The listing builds one solid part. Answer for the finished solid, in the listing's coordinates (mm). A direction names the side the tool comes from. Coordinates: 2 decimals unless noted, no trailing zeros. Order: outer loops, then holes, each group sorted by start corner. A loop starts at its lowest first (then second) coordinate and runs counter-clockwise, first axis right, second up. Notation, with made-up numbers: (32.5, 55.5) -> (85.5, 55.5) arc R26 ccw to (85.5, 93.5) -> close; hole circle Ø1 at (43, 2). An arc over 180 degrees is marked (long way). Return JSON: item names as keys, results as strings.
```python
from build123d import *

# Parameters (mm, degrees)
EXTRUDE_1_OUTLINE_R   = 35
EXTRUDE_1_OUTLINE_R_2 = 1.55
EXTRUDE_1_OUTLINE_R_3 = 30.05
EXTRUDE_1_DEPTH       = 10
SKETCH_2_R            = 33.525
SKETCH_2_R_2          = 18.525
EXTRUDE_1_2_DEPTH     = 4
SKETCH_3_R            = 1.55
CUT_EXTRUDE_1_DEPTH   = 51.497524692
CUT_EXTRUDE_2_DEPTH   = 6
SKETCH_8_R            = 35
SKETCH_8_R_2          = 30.05
CUT_EXTRUDE_3_DEPTH   = 2
SKETCH_9_R            = 3
CUT_EXTRUDE_4_DEPTH   = 2
SKETCH_10_R           = 1.55
CUT_EXTRUDE_5_DEPTH   = 51.139804547
SKETCH_11_R           = 3
CUT_EXTRUDE_6_DEPTH   = 2
SKETCH_14_R           = 18.525
SKETCH_14_R_2         = 13.5
EXTRUDE_2_DEPTH       = 4
SKETCH_15_R           = 17.5
CUT_EXTRUDE_8_DEPTH   = 1
SKETCH_17_R           = 17.5
SKETCH_17_R_2         = 12.5
CUT_EXTRUDE_9_DEPTH   = 1
SKETCH1_R             = 13.5
SKETCH1_R_2           = 12
BOSS_EXTRUDE1_DEPTH   = 1
SKETCH2_R             = 12.5
SKETCH2_R_2           = 12
CUT_EXTRUDE1_DEPTH    = 50.989999


# Read off the part's stored shape, not the designer's step: 凸台-拉伸1
with BuildPart() as part:
    # Extrude 1 outline → Extrude 1 (new body)
    with BuildSketch(Plane.XY):
        Circle(EXTRUDE_1_OUTLINE_R)
        with Locations((0, -32.5)):
            Circle(EXTRUDE_1_OUTLINE_R_2, mode=Mode.SUBTRACT)
        with Locations((-32.5, 0)):
            Circle(EXTRUDE_1_OUTLINE_R_2, mode=Mode.SUBTRACT)
        Circle(EXTRUDE_1_OUTLINE_R_3, mode=Mode.SUBTRACT)
        with Locations((32.5, 0)):
            Circle(EXTRUDE_1_OUTLINE_R_2, mode=Mode.SUBTRACT)
        with Locations((0, 32.5)):
            Circle(EXTRUDE_1_OUTLINE_R_2, mode=Mode.SUBTRACT)
    extrude(amount=EXTRUDE_1_DEPTH)

    # 草图2 → Extrude 1 2 (add)
    with BuildSketch(Plane.XY.offset(10)):
        Circle(SKETCH_2_R)
        Circle(SKETCH_2_R_2, mode=Mode.SUBTRACT)
    extrude(amount=-EXTRUDE_1_2_DEPTH)

    # 草图3 → 切除-拉伸1 (cut, through all)
    with BuildSketch(Plane(origin=(0, 0, 0), x_dir=(-1, 0, 0), z_dir=(0, 0, -1))):
        with Locations(Location((32.5, 0, 0), (0, 0, 180))):
            Circle(SKETCH_3_R)
        with Locations(Location((0, -32.5, 0), (0, 0, 180))):
            Circle(SKETCH_3_R)
        with Locations(Location((-32.5, 0, 0), (0, 0, 180))):
            Circle(SKETCH_3_R)
        with Locations(Location((0, 32.5, 0), (0, 0, 180))):
            Circle(SKETCH_3_R)
    extrude(amount=-CUT_EXTRUDE_1_DEPTH, mode=Mode.SUBTRACT)

    # 草图7 → 切除-拉伸2 (cut)
    with BuildSketch(Plane(origin=(0, 0, 0), x_dir=(-1, 0, 0), z_dir=(0, 0, -1))):
        with BuildLine():
            Line((15.025, 26.024063384), (17.5, 30.310889132))
            ThreePointArc((17.5, 30.310889132), (24.748737342, 24.748737342), (30.310889132, 17.5))
            Line((30.310889132, 17.5), (26.024063384, 15.025))
            ThreePointArc((26.024063384, 15.025), (21.248558775, 21.248558775), (15.025, 26.024063384))
        make_face()
    extrude(amount=-CUT_EXTRUDE_2_DEPTH, mode=Mode.SUBTRACT)

    # 草图8 → 切除-拉伸3 (cut)
    with BuildSketch(Plane(origin=(0, 0, 0), x_dir=(-1, 0, 0), z_dir=(0, 0, -1))):
        with Locations(Location((0, 0, 0), (0, 0, 30))):
            Circle(SKETCH_8_R)
        Circle(SKETCH_8_R_2, mode=Mode.SUBTRACT)
    extrude(amount=-CUT_EXTRUDE_3_DEPTH, mode=Mode.SUBTRACT)

    # 草图9 → 切除-拉伸4 (cut)
    with BuildSketch(Plane.XY.offset(10)):
        with Locations((0, 32.5)):
            Circle(SKETCH_9_R)
        with Locations((32.5, 0)):
            Circle(SKETCH_9_R)
        with Locations((0, -32.5)):
            Circle(SKETCH_9_R)
        with Locations((-32.5, 0)):
            Circle(SKETCH_9_R)
    extrude(amount=-CUT_EXTRUDE_4_DEPTH, mode=Mode.SUBTRACT)

    # 草图10 → 切除-拉伸5 (cut, through all)
    with BuildSketch(Plane.XY.offset(10)):
        with Locations((22.980970389, 22.980970389)):
            Circle(SKETCH_10_R)
        with Locations((22.980970389, -22.980970389)):
            Circle(SKETCH_10_R)
        with Locations((-22.980970389, -22.980970389)):
            Circle(SKETCH_10_R)
        with Locations((-22.980970389, 22.980970389)):
            Circle(SKETCH_10_R)
    extrude(amount=-CUT_EXTRUDE_5_DEPTH, mode=Mode.SUBTRACT)

    # 草图11 → 切除-拉伸6 (cut)
    with BuildSketch(Plane.XY.offset(10)):
        with Locations((22.980970389, 22.980970389)):
            Circle(SKETCH_11_R)
        with Locations((22.980970389, -22.980970389)):
            Circle(SKETCH_11_R)
        with Locations((-22.980970389, -22.980970389)):
            Circle(SKETCH_11_R)
        with Locations((-22.980970389, 22.980970389)):
            Circle(SKETCH_11_R)
    extrude(amount=-CUT_EXTRUDE_6_DEPTH, mode=Mode.SUBTRACT)

    # 草图14 → 凸台-拉伸2 (add)
    with BuildSketch(Plane.XY.offset(10)):
        Circle(SKETCH_14_R)
        Circle(SKETCH_14_R_2, mode=Mode.SUBTRACT)
    extrude(amount=-EXTRUDE_2_DEPTH)

    # 草图15 → 切除-拉伸8 (cut)
    with BuildSketch(Plane.XY.offset(10)):
        with BuildLine():
            ThreePointArc((21.378493867, 1.75), (0, 21.45), (-21.378493867, 1.75))
            Line((-21.378493866, 1.75), (-24.8, 1.75))
            Line((-24.8, 1.75), (-24.8, -1.75))
            Line((-24.8, -1.75), (-21.378493867, -1.75))
            ThreePointArc((-21.378493867, -1.75), (0, -21.45), (21.378493867, -1.75))
            Line((21.378493867, -1.75), (24.8, -1.75))
            Line((24.8, -1.75), (24.8, 1.75))
            Line((24.8, 1.75), (21.378493867, 1.75))
        make_face()
        Circle(SKETCH_15_R, mode=Mode.SUBTRACT)
    extrude(amount=-CUT_EXTRUDE_8_DEPTH, mode=Mode.SUBTRACT)

    # 草图17 → 切除-拉伸9 (cut)
    with BuildSketch(Plane.XY.offset(10)):
        Circle(SKETCH_17_R)
        Circle(SKETCH_17_R_2, mode=Mode.SUBTRACT)
    extrude(amount=-CUT_EXTRUDE_9_DEPTH, mode=Mode.SUBTRACT)

    # Sketch1 → Boss-Extrude1 (add)
    with BuildSketch(Plane.XY.offset(9)):
        Circle(SKETCH1_R)
        Circle(SKETCH1_R_2, mode=Mode.SUBTRACT)
    extrude(amount=-BOSS_EXTRUDE1_DEPTH)

    # Sketch2 → Cut-Extrude1 (cut, through all)
    with BuildSketch(Plane.XY.offset(9)):
        Circle(SKETCH2_R)
        Circle(SKETCH2_R_2, mode=Mode.SUBTRACT)
    extrude(amount=-CUT_EXTRUDE1_DEPTH, mode=Mode.SUBTRACT)


solid = part.part
```
Item 1: Flat-ended cylindrical pins translate along their axes: pin 1 (4 mm diameter, centred on x = -22, y = 15.5, fed in from -Z); pin 2 (16 mm diameter, centred on x = 0, y = 0, fed in from -Z); pin 3 (5.5 mm diameter, centred on x = 32.5, y = 0, fed in from +Z); pin 4 (0.8 mm diameter, centred on x = -22.5, z = 9.5, fed in from -Y). Find the tip coordinate at first contact, or state that the pin passes through.
Answer list:
{"pin 1": "z = 6", "pin 2": "through", "pin 3": "z = 8", "pin 4": "y = -27.14"}
Item 2: Find the intervals of material crossed by probe 1 along Y at (x, z) = (0, 4.25); probe 2 along Z at (x, y) = (23.5, 12); probe 3 along Z at (x, y) = (15.5, 10), in increasing order.
Answer list:
{"probe 1": "-35 to -34.05, -30.95 to -30.05, 30.05 to 30.95, 34.05 to 35", "probe 2": "6 to 10", "probe 3": "6 to 9"}
Item 3: Determine the mould class of faces 4 (the cylindrical face through (20.936, -20.786, 9.014)), 5 (the flat face through (1, 31, 8)), 6 (the flat face through (14.9, -26.4, 2)) for opening direction Z: pulls with the +Z half, pulls with the -Z half, needs draft (parallel to the pull), parting line crosses it, or undercut.
Answer list:
{"face 4": "needs draft", "face 5": "pulls with the +Z half", "face 6": "pulls with the -Z half"}
Item 4: The part is cut by section A-A on x = 0. Count the separate pieces of the cut face and the enclosed holes in it, plus the area to 4 significant figures.
Answer list:
{"separate pieces": "4", "enclosed holes": "0", "area": "138.5 mm2"}
Item 5: The part is cut by section B-B on x = -32.5. Determine the outline of the cut face in (y, z).
Answer list:
{"outline": "(-12.99, 2) -> (-1.55, 2) -> (-1.55, 8) -> (-3, 8) -> (-3, 10) -> (-12.99, 10) -> close; (1.55, 2) -> (12.99, 2) -> (12.99, 10) -> (3, 10) -> (3, 8) -> (1.55, 8) -> close"}
Item 6: The part is cut by section D-D on z = 4.75. Determine the outline of the cut face in (x, y) (3 decimals), plus the area to 3 significant figures.
Answer list:
{"outline": "(-30.311, 17.5) arc R35 ccw (long way) to (-17.5, 30.311) -> (-15.025, 26.024) arc R30.05 cw (long way) to (-26.024, 15.025) -> close; hole circle Ø3.1 at (-32.5, 0); hole circle Ø3.1 at (-22.981, -22.981); hole circle Ø3.1 at (0, -32.5); hole circle Ø3.1 at (0, 32.5); hole circle Ø3.1 at (22.981, -22.981); hole circle Ø3.1 at (22.981, 22.981); hole circle Ø3.1 at (32.5, 0)", "area": "874 mm2"}
Item 7: Which of the six approach directions +Z, -Z, +X, -X, +Y, -Y give full straight-line access (tool end or side, diameter ignored) to faces 1 (the cylindrical face through (11.923, 3.755, 8.507)), 2 (the flat face through (1, -31, 8)), 3 (the flat face through (-16.245, 28.137, 3.972))?
Answer list:
{"face 1": "+Z, -Z", "face 2": "+Z", "face 3": "-Z, -X"}
